from build123d import *

# Parameters (mm, degrees)
F0_R     = 4.953
F1_DEPTH = 12.192
F2_DEPTH = 45.974
F4_DEPTH = 203.2


with BuildPart() as f1:
    # F0 (on Front) → F1 (new body)
    with BuildSketch(Plane.XZ):
        with BuildLine():
            Line((50.8, 0), (12.7, 0))
            ThreePointArc((12.7, 0), (3.7197438789, -3.7197438789), (0, -12.7))
            Line((0, -12.7), (0, -76.2))
            ThreePointArc((0, -76.2), (3.7197438789, -85.1802561211), (12.7, -88.9))
            Line((12.7, -88.9), (50.8, -88.9))
            ThreePointArc((50.8, -88.9), (59.7802561211, -85.1802561211), (63.5, -76.2))
            Line((63.5, -76.2), (63.5, -12.7))
            ThreePointArc((63.5, -12.7), (59.7802561211, -3.7197438789), (50.8, 0))
        make_face()
        with Locations((12.7, -76.2)):
            Circle(F0_R, mode=Mode.SUBTRACT)
        Polygon((31.0494050882, -19.2913363232), (33.909, -17.6403), (56.134, -56.134), (53.2744050882, -57.7850363232), (45.1355580316, -62.4841397046), (39.6363370474, -65.6592095569), (31.4974899908, -70.3583129383), (28.637895079, -72.0093492615), (6.412895079, -33.5156492615), (9.2724899908, -31.8646129383), (17.4113370474, -27.1655095569), (22.9105580316, -23.9904397046), align=None, mode=Mode.SUBTRACT)
        with Locations((50.8, -76.2)):
            Circle(F0_R, mode=Mode.SUBTRACT)
        with Locations((12.7, -12.7)):
            Circle(F0_R, mode=Mode.SUBTRACT)
        with Locations((50.8, -12.7)):
            Circle(F0_R, mode=Mode.SUBTRACT)
    extrude(amount=F1_DEPTH)

    # F0 (on Front) → F2 (join)
    with BuildSketch(Plane.XZ):
        Polygon((56.134, -56.134), (33.909, -17.6403), (31.0494050882, -19.2913363232), (53.2744050882, -57.7850363232), align=None)
        Polygon((53.2744050882, -57.7850363232), (31.0494050882, -19.2913363232), (22.9105580316, -23.9904397046), (45.1355580316, -62.4841397046), align=None)
        Polygon((45.1355580316, -62.4841397046), (22.9105580316, -23.9904397046), (17.4113370474, -27.1655095569), (39.6363370474, -65.6592095569), align=None)
        Polygon((39.6363370474, -65.6592095569), (17.4113370474, -27.1655095569), (9.2724899908, -31.8646129383), (31.4974899908, -70.3583129383), align=None)
        Polygon((31.4974899908, -70.3583129383), (9.2724899908, -31.8646129383), (6.412895079, -33.5156492615), (28.637895079, -72.0093492615), align=None)
    extrude(amount=F2_DEPTH)

    # F3 (on face) → F4 (cut)
    with BuildSketch(Plane(origin=(38.3412090132, 0, -66.4069740109), x_dir=(0.8660190526, 0, 0.5000110004), z_dir=(0.5000110004, 0, -0.8660190526))):
        Polygon((-7.9025039941, 45.974), (1.4954960059, 32.004), (1.4954960059, 26.924), (7.8454960059, 26.924), (7.8454960059, 32.004), (17.2434960059, 45.974), align=None)
    extrude(amount=-F4_DEPTH, mode=Mode.SUBTRACT)


solid = f1.part
Geometry check sheet. Reference: the model listing, model coordinates, mm. A direction names the side the tool comes from. Round coordinates to 2 decimals unless told otherwise and drop trailing zeros. Write each loop counter-clockwise with the first axis right and the second up, starting at its lowest first coordinate (ties: lowest second). Pieces come first, ordered by that corner, then holes.
Item 1: Go/stop test with flat-tipped pins: pin 1 Ø13 at (x, z) = (12.7, -12.7) entering from +Y; pin 2 Ø5 at (x, z) = (53, -43.5) entering from -Y; pin 3 Ø12 at (x, y) = (24.5, -35.5) entering from +Z; pin 4 Ø8 at (y, z) = (-28, -66.5) entering from -X. Record where each tip stops, or that it passes through.
Determined:
pin 1: stops at y = 0
pin 2: stops at y = -12.19
pin 3: stops at z = -19.61
pin 4: stops at x = 23.15
Item 2: Material ranges on line 1 along Z through (x, y) = (50.8, -7.5); line 2 along X through (y, z) = (-5, -76), recorded low to high.
Determined:
line 1: z = -88.9 to -81.15, -71.25 to -17.65, -7.75 to 0
line 2: x = 0 to 7.75, 17.65 to 45.85, 55.75 to 63.5
Item 3: Section check D-D (z = -30). Record the boundary of the cut face in (x, y), plus the area to 3 significant figures.
Determined:
outline: (0, -12.19) - (12.5, -12.19) - (12.5, -40.43) - (19.05, -32) - (19.05, -26.92) - (26.38, -26.92) - (26.38, -32) - (37.23, -45.97) - (41.05, -45.97) - (41.05, -12.19) - (63.5, -12.19) - (63.5, 0) - (0, 0) - close
area: 1,460 mm2
Item 4: Mould release check, pull along X, two halves, no side actions. Record for faces 1 (the face through (3.82, -6.01, -3.62)), 2 (the face through (31, -6, -88.9)), 3 (the face through (59.88, -6.01, -3.82)), 4 (the face through (14.99, -6.01, -17.09)): +X half, -X half, draft (parallel to the pull), parting line (faces both ways), or undercut.
Determined:
face 1: -X half
face 2: draft
face 3: +X half
face 4: undercut
Item 5: Section check A-A (z = -16.5). Record the boundary of the cut face in (x, y).
Determined:
outline: (0, -12.19) - (9.52, -12.19) - (9.52, 0) - (0, 0) - close; (15.88, -12.19) - (47.62, -12.19) - (47.62, 0) - (15.88, 0) - close; (53.98, -12.19) - (63.5, -12.19) - (63.5, 0) - (53.98, 0) - close
Item 6: Access from +Z, -Z, +X, -X, +Y, -Y to the whole of each face (thin tool, end or side, straight path). Record for faces 5 (the face through (34.18, -29.43, -43.51)), 6 (the face through (45.2, -28.8, -37.2)), 7 (the face through (17.37, -28.85, -52.49)).
Determined:
face 5: -Y
face 6: +Z, +X, -Y
face 7: -Z, -X, -Y
Item 7: Section check C-C (y = -6.5). Record the boundary of the cut face in (x, z), plus the area to 3 significant figures.
Determined:
outline: (0, -76.2) arc R12.7 ccw to (12.7, -88.9) - (50.8, -88.9) arc R12.7 ccw to (63.5, -76.2) - (63.5, -12.7) arc R12.7 ccw to (50.8, 0) - (12.7, 0) arc R12.7 ccw to (0, -12.7) - close; hole circle Ø9.91 at (12.7, -76.2); hole circle Ø9.91 at (12.7, -12.7); hole circle Ø9.91 at (50.8, -76.2); hole circle Ø9.91 at (50.8, -12.7)
area: 5,200 mm2
Item 8: Section check B-B (y = -16.5). Record the boundary of the cut face in (x, z), plus the area to 3 significant figures.
Determined:
outline: (6.41, -33.52) - (28.64, -72.01) - (56.13, -56.13) - (33.91, -17.64) - close
area: 1,410 mm2
